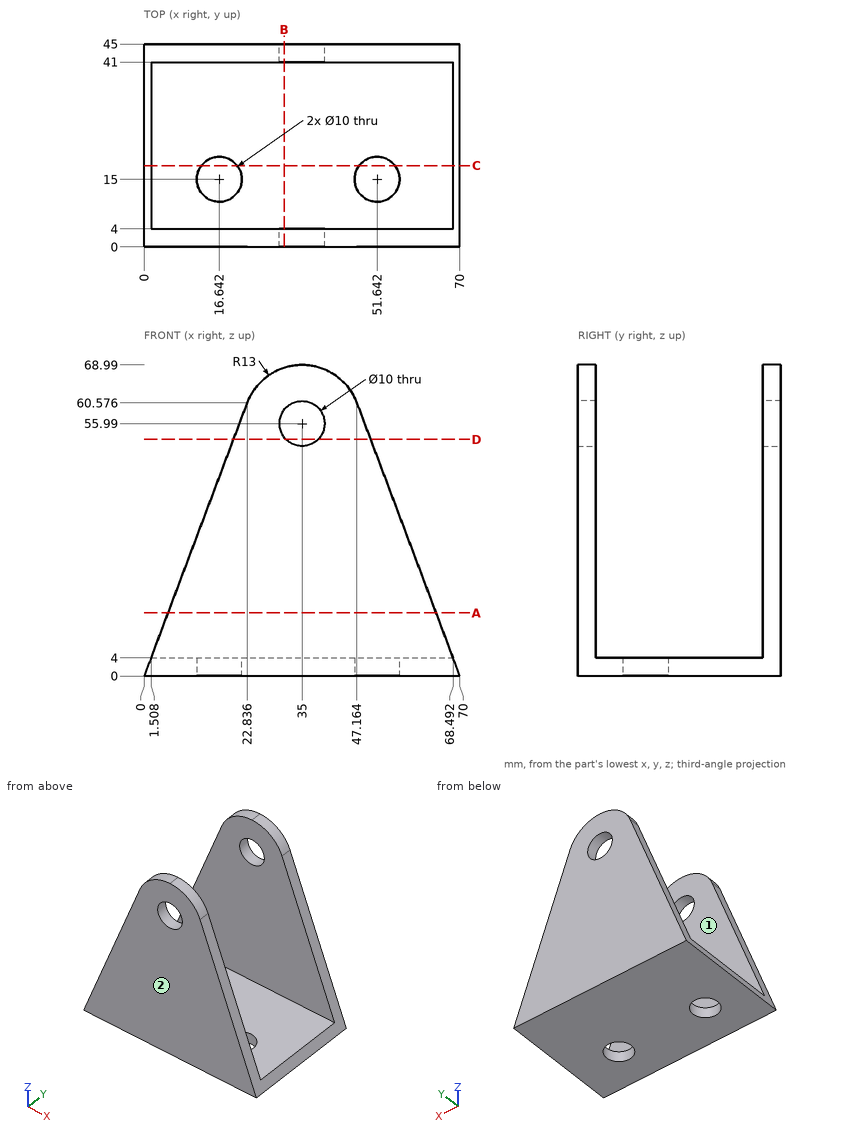
Study the drawing (mm; zero at the part's minimum x, y, z) and answer. A direction names the side the tool comes from. Round coordinates to 2 decimals unless told otherwise and drop trailing zeros. Write each loop counter-clockwise with the first axis right and the second up, starting at its lowest first coordinate (ties: lowest second). Pieces come first, ordered by that corner, then holes.
Q1. Find section A-A on z = 14. Determine the outline of the cut face in (x, y).
Values:
outline: (5.28, 0) - (64.72, 0) - (64.72, 4) - (5.28, 4) - close; (5.28, 41) - (64.72, 41) - (64.72, 45) - (5.28, 45) - close
Q2. Find section B-B on x = 31. Determine the outline of the cut face in (y, z).
Values:
outline: (0, 0) - (45, 0) - (45, 52.99) - (41, 52.99) - (41, 4) - (4, 4) - (4, 52.99) - (0, 52.99) - close; (0, 58.99) - (4, 58.99) - (4, 68.36) - (0, 68.36) - close; (41, 58.99) - (45, 58.99) - (45, 68.36) - (41, 68.36) - close
Q3. Find section D-D on z = 52.5. Determine the outline of the cut face in (x, y).
Values:
outline: (19.79, 0) - (31.42, 0) - (31.42, 4) - (19.79, 4) - close; (19.79, 41) - (31.42, 41) - (31.42, 45) - (19.79, 45) - close; (38.58, 0) - (50.21, 0) - (50.21, 4) - (38.58, 4) - close; (38.58, 41) - (50.21, 41) - (50.21, 45) - (38.58, 45) - close
Q4. A tool of negligible diameter and unlimited length cuts with its end or side. For the marked faces 1 and 2, from which of +Z, -Z, +X, -X, +Y, -Y can it reach the whole face along a straight path? Write none if from no direction.
Values:
face 1: +Z, +X, -X
face 2: +Z, -Z, +X, -X, -Y
Q5. Straight lines are drawn through the part: line 1 (Y direction, x = 35, z = 8.5); line 2 (Z direction, x = 9, y = 10); line 3 (X direction, y = 3.5, z = 28.5) (1 decimal). For each, find the intervals that lie inside material, in ascending order.
Values:
line 1: y = 0 to 4, 41 to 45
line 2: z = 0 to 4
line 3: x = 10.7 to 59.3
Q6. Find section C-C on y = 18. Determine the outline of the cut face in (x, z), and give its area (3 significant figures).
Values:
outline: (0, 0) - (12.64, 0) - (12.64, 4) - (1.51, 4) - close; (20.64, 0) - (47.64, 0) - (47.64, 4) - (20.64, 4) - close; (55.64, 0) - (70, 0) - (68.49, 4) - (55.64, 4) - close
area: 210 mm2
Q7. Flat-ended cylindrical pins translate along their axes: P1, Ø3, axis at x = 28.5, y = 36, coming from the +Z side; P2, Ø16, axis at x = 51.64, y = 15, coming from the -Z side; P3, Ø4, axis at x = 44.5, y = 40.5, coming from the +Z side; P4, Ø6, axis at x = 35, z = 55.99, coming from the +Y side. Find the tip coordinate at first contact, or state that the pin passes through.
Values:
P1: stops at z = 4
P2: stops at z = 0
P3: stops at z = 66.56
P4: passes through
